For this review, take the finished solid that the model builds, in its own axes (mm). A direction names the side the tool comes from. Give positions to 0.01 mm unless a question says otherwise; leave off trailing zeros. Loops run counter-clockwise (first coordinate to the right, second up) from the corner with the lowest first, then second, coordinate; pieces in that order, holes last. Notation, with made-up numbers: (59.5, -10.5) -> (68.5, -10.5) arc R25 ccw to (68.5, 3.5) -> close; hole circle Ø5 at (-33, 6). An arc over 180 degrees is marked (long way). Answer as CSV lines item,"result". Start each with the question number.
Item 1: Clearance check with a flat-ended pin moving along its axis: P1, Ø2, axis at y = -12.5, z = 6.5, coming from the -X side. State where the tip first meets the part, or that it passes through.
Item 2: Add section D-D on z = 12.7. State the section outline as (x, y) points (3 decimals), plus the area to 3 significant figures.
Item 3: Add section B-B on x = 6. State the section outline as (y, z) points, plus the area to 3 significant figures.
Item 4: For L1, parallel to Y at x = 13, z = 4.25; L2, parallel to X at y = -16.75, z = 6.5; L3, parallel to X at y = -4.75, z = 10, list the stretches that pass through material, from the lowest coordinate up. Write a range as from..to.
Item 5: Add section C-C on y = -13.97. State the section outline as (x, z) points (3 decimals).
Item 6: Add section A-A on z = 2.5. State the section outline as (x, y) points.
Item 7: Machinability: for faces 1 (the face through (88, 0, 13)), 2 (the face through (2.25, -14.85, 11.01)), 3 (the face through (24.384, -14, 13)), which of the approach directions +Z, -Z, +X, -X, +Y, -Y give a long, thin tool a straight path to every point of the face, cutting with its end or side? Answer none if there is none.
Item 8: The part is to be moulded in two halves that separate along X. For faces 4 (the face through (44, -14, 0)), 5 (the face through (0, -14, 15)), 6 (the face through (81.688, -5.567, 12.522)), say which applies: +X half, -X half, draft (parallel to the pull), parting line (faces both ways), or undercut.
```python
from build123d import *

# Parameters (mm, degrees)
F0_W     = 19.812
F0_H     = 19.05
F1_DEPTH = 25.4
F2_R     = 1.905
F3_DEPTH = 7.62


with BuildPart() as f1:
    # F0 (on Top) → F1 (new body)
    with BuildSketch(Plane.XY):
        with BuildLine():
            Line((78.070664, 0), (0, 0))
            Line((0, 0), (0, -27.94))
            Line((0, -27.94), (88.9, -27.94))
            Line((88.9, -27.94), (88.9, 0))
            Line((88.9, 0), (86.36, 0))
            Line((86.36, 0), (76.884093, -11.292947))
            ThreePointArc((76.884093, -11.292947), (72.378782, -11.315446), (72.356282, -6.810135))
            Line((72.356282, -6.810135), (78.070664, 0))
        make_face()
        with Locations((14.478, -13.843)):
            Rectangle(F0_W, F0_H, mode=Mode.SUBTRACT)
    extrude(amount=F1_DEPTH)

    # F2 (on face) → F3 (cut)
    with BuildSketch(Plane(origin=(0, 0, 0), x_dir=(0, -1, 0), z_dir=(-1, 0, 0))):
        with Locations((13.97, 12.7)):
            Circle(F2_R)
    extrude(amount=-F3_DEPTH, mode=Mode.SUBTRACT)


solid = f1.part
```
Computed values:
1,P1,"x = 0"
2,outline,"(0, -27.94) -> (88.9, -27.94) -> (88.9, 0) -> (86.36, 0) -> (76.884, -11.293) arc R3.186 cw to (72.356, -6.81) -> (78.071, 0) -> (0, 0) -> (0, -12.065) -> (4.572, -12.065) -> (4.572, -4.318) -> (24.384, -4.318) -> (24.384, -23.368) -> (4.572, -23.368) -> (4.572, -15.875) -> (0, -15.875) -> close"
2,area,"2,000 mm²"
3,outline,"(-27.94, 0) -> (-23.37, 0) -> (-23.37, 25.4) -> (-27.94, 25.4) -> close; (-4.32, 0) -> (0, 0) -> (0, 25.4) -> (-4.32, 25.4) -> close"
3,area,"226 mm²"
4,L1,"-27.94..-23.37, -4.32..0"
4,L2,"0..4.57, 24.38..88.9"
4,L3,"0..4.57, 24.38..74.08, 82.37..88.9"
5,outline,"(0, 0) -> (4.572, 0) -> (4.572, 10.795) -> (0, 10.795) -> close; (0, 14.605) -> (4.572, 14.605) -> (4.572, 25.4) -> (0, 25.4) -> close; (24.384, 0) -> (88.9, 0) -> (88.9, 25.4) -> (24.384, 25.4) -> close"
6,outline,"(0, -27.94) -> (88.9, -27.94) -> (88.9, 0) -> (86.36, 0) -> (76.88, -11.29) arc R3.19 cw to (72.36, -6.81) -> (78.07, 0) -> (0, 0) -> close; hole (4.57, -23.37) -> (24.38, -23.37) -> (24.38, -4.32) -> (4.57, -4.32) -> close"
7,face 1,"+Z, -Z, +X, -X, +Y"
7,face 2,"-X"
7,face 3,"+Z, -Z"
8,face 4,"draft"
8,face 5,"-X half"
8,face 6,"undercut"
